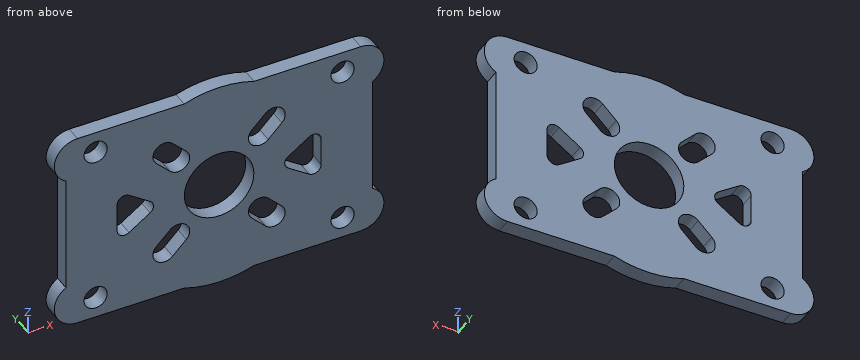
from build123d import *

# Parameters (mm, degrees)
SKETCH1_R           = 1.5
SKETCH1_R_2         = 4.5
BOSS_EXTRUDE1_DEPTH = 2


with BuildPart() as part:
    # Sketch1 → Boss-Extrude1 (new body)
    with BuildSketch(Plane(origin=(0, 0, 0), x_dir=(1, 0, 0), z_dir=(0, 1, 0))):
        with BuildLine():
            Line((-18.35, -13.3), (-4.529072753, -13.3))
            ThreePointArc((-4.529072753, -13.3), (0, -14.05), (4.529072753, -13.3))
            Line((4.529072753, -13.3), (18.35, -13.3))
            ThreePointArc((18.35, -13.3), (21.247777479, -11.076457135), (19.85, -7.701923789))
            Line((19.85, -7.701923789), (19.85, 7.701923789))
            ThreePointArc((19.85, 7.701923789), (21.247777479, 11.076457135), (18.35, 13.3))
            Line((18.35, 13.3), (4.529072753, 13.3))
            ThreePointArc((4.529072753, 13.3), (0, 14.05), (-4.529072753, 13.3))
            Line((-4.529072753, 13.3), (-18.35, 13.3))
            ThreePointArc((-18.35, 13.3), (-21.247777479, 11.076457135), (-19.85, 7.701923789))
            Line((-19.85, 7.701923789), (-19.85, -7.701923789))
            ThreePointArc((-19.85, -7.701923789), (-21.247777479, -11.076457135), (-18.35, -13.3))
        make_face()
        with Locations(Location((-16, 10.5, 0), (0, 0, 270))):
            Circle(SKETCH1_R, mode=Mode.SUBTRACT)
        with Locations(Location((-16, -10.5, 0), (0, 0, 270))):
            Circle(SKETCH1_R, mode=Mode.SUBTRACT)
        with Locations(Location((16, -10.5, 0), (0, 0, 270))):
            Circle(SKETCH1_R, mode=Mode.SUBTRACT)
        with Locations(Location((16, 10.5, 0), (0, 0, 270))):
            Circle(SKETCH1_R, mode=Mode.SUBTRACT)
        with Locations(Location((0, 0, 0), (0, 0, 270))):
            Circle(SKETCH1_R_2, mode=Mode.SUBTRACT)
        with BuildLine():
            Line((-6.01040764, 8.131727984), (-4.242640687, 6.363961031))
            ThreePointArc((-4.242640687, 6.363961031), (-4.242640687, 4.242640687), (-6.363961031, 4.242640687))
            Line((-6.363961031, 4.242640687), (-8.131727984, 6.01040764))
            ThreePointArc((-8.131727984, 6.01040764), (-8.131727984, 8.131727984), (-6.01040764, 8.131727984))
        make_face(mode=Mode.SUBTRACT)
        with BuildLine():
            Line((8.131727984, 6.01040764), (6.363961031, 4.242640687))
            ThreePointArc((6.363961031, 4.242640687), (4.242640687, 4.242640687), (4.242640687, 6.363961031))
            Line((4.242640687, 6.363961031), (6.01040764, 8.131727984))
            ThreePointArc((6.01040764, 8.131727984), (8.131727984, 8.131727984), (8.131727984, 6.01040764))
        make_face(mode=Mode.SUBTRACT)
        with BuildLine():
            Line((6.01040764, -8.131727984), (4.242640687, -6.363961031))
            ThreePointArc((4.242640687, -6.363961031), (4.242640687, -4.242640687), (6.363961031, -4.242640687))
            Line((6.363961031, -4.242640687), (8.131727984, -6.01040764))
            ThreePointArc((8.131727984, -6.01040764), (8.131727984, -8.131727984), (6.01040764, -8.131727984))
        make_face(mode=Mode.SUBTRACT)
        with BuildLine():
            Line((-8.131727984, -6.01040764), (-6.363961031, -4.242640687))
            ThreePointArc((-6.363961031, -4.242640687), (-4.242640687, -4.242640687), (-4.242640687, -6.363961031))
            Line((-4.242640687, -6.363961031), (-6.01040764, -8.131727984))
            ThreePointArc((-6.01040764, -8.131727984), (-8.131727984, -8.131727984), (-8.131727984, -6.01040764))
        make_face(mode=Mode.SUBTRACT)
        with BuildLine():
            Line((-13.224863073, 1.857861186), (-13.224863073, -1.857861186))
            ThreePointArc((-13.224863073, -1.857861186), (-12.69212273, -2.74198132), (-11.661526248, -2.684088529))
            Line((-11.661526248, -2.684088529), (-8.936663175, -0.826227343))
            ThreePointArc((-8.936663175, -0.826227343), (-8.5, 0), (-8.936663175, 0.826227343))
            Line((-8.936663175, 0.826227343), (-11.661526248, 2.684088529))
            ThreePointArc((-11.661526248, 2.684088529), (-12.69212273, 2.74198132), (-13.224863073, 1.857861186))
        make_face(mode=Mode.SUBTRACT)
        with BuildLine():
            Line((11.661526248, -2.684088529), (8.936663175, -0.826227343))
            ThreePointArc((8.936663175, -0.826227343), (8.5, 0), (8.936663175, 0.826227343))
            Line((8.936663175, 0.826227343), (11.661526248, 2.684088529))
            ThreePointArc((11.661526248, 2.684088529), (12.69212273, 2.74198132), (13.224863073, 1.857861186))
            Line((13.224863073, 1.857861186), (13.224863073, -1.857861186))
            ThreePointArc((13.224863073, -1.857861186), (12.69212273, -2.74198132), (11.661526248, -2.684088529))
        make_face(mode=Mode.SUBTRACT)
    extrude(amount=BOSS_EXTRUDE1_DEPTH)


solid = part.part
The model under review builds one solid part; all positions refer to its coordinate system, in mm. Give positions to 0.01 mm unless a question says otherwise; leave off trailing zeros. Loops run counter-clockwise (first coordinate to the right, second up) from the corner with the lowest first, then second, coordinate; pieces in that order, holes last. Notation, with made-up numbers: (28.25, -23) -> (52.25, -23) arc R27 cw to (52.25, 15) -> close; hole circle Ø1 at (42.5, 89.5). An arc over 180 degrees is marked (long way). Answer as a JSON object with one key per item and string values. Group by question number.
Q1. Take a section at A-A (x = 0). Write out the cut boundary in (y, z).
Q2. Take a section at B-B (x = 16). Write out the cut boundary in (y, z).
Q3. Take a section at C-C (z = 0). Write out the cut boundary in (x, y).
Q4. Insertion check: pin 1 (2 mm diameter, centred on x = 0.5, z = -3.5, fed in from -Y); pin 2 (2.5 mm diameter, centred on x = 16, z = -10.5, fed in from -Y); pin 3 (0.6 mm diameter, centred on y = 1, z = -2.5, fed in from -X); pin 4 (1 mm diameter, centred on x = -11, y = 1.5, fed in from -Z). Each pin has a flat end and moves straight along its axis. Give the tip position at first contact, or say it passes through.
Q5. Take a section at D-D (z = -10.5). Write out the cut boundary in (x, y), plus the area to 3 significant figures.
Q6. Wall thickness on line 1 along X through (y, z) = (0.55, 10.5); line 2 along X through (y, z) = (1.1, -0.5); line 3 along X through (y, z) = (0.6, -4.75): over which ranges is each line inside the solid? List them lowest first.
Answer below:
{
 "1": {"outline": "(0, -14.05) -> (2, -14.05) -> (2, -4.5) -> (0, -4.5) -> close; (0, 4.5) -> (2, 4.5) -> (2, 14.05) -> (0, 14.05) -> close"},
 "2": {"outline": "(0, -13.3) -> (2, -13.3) -> (2, -12) -> (0, -12) -> close; (0, -9) -> (2, -9) -> (2, 9) -> (0, 9) -> close; (0, 12) -> (2, 12) -> (2, 13.3) -> (0, 13.3) -> close"},
 "3": {"outline": "(-19.85, 0) -> (-13.22, 0) -> (-13.22, 2) -> (-19.85, 2) -> close; (-8.5, 0) -> (-4.5, 0) -> (-4.5, 2) -> (-8.5, 2) -> close; (4.5, 0) -> (8.5, 0) -> (8.5, 2) -> (4.5, 2) -> close; (13.22, 0) -> (19.85, 0) -> (19.85, 2) -> (13.22, 2) -> close"},
 "4": {"pin 1": "stops at y = 0", "pin 2": "passes through", "pin 3": "stops at x = -19.85", "pin 4": "stops at z = -13.3"},
 "5": {"outline": "(-21.34, 0) -> (-17.5, 0) -> (-17.5, 2) -> (-21.34, 2) -> close; (-14.5, 0) -> (14.5, 0) -> (14.5, 2) -> (-14.5, 2) -> close; (17.5, 0) -> (21.34, 0) -> (21.34, 2) -> (17.5, 2) -> close", "area": "73.4 mm2"},
 "6": {"line 1": "x = -21.34 to -17.5, -14.5 to 14.5, 17.5 to 21.34", "line 2": "x = -19.85 to -13.22, -8.63 to -4.47, 4.47 to 8.63, 13.22 to 19.85", "line 3": "x = -19.85 to -6.87, -3.91 to 3.91, 6.87 to 19.85"}
}
